from build123d import *

# Parameters (mm, degrees)
F0_W     = 0.75
F0_H     = 2
F1_DEPTH = 12
F2_W     = 6.62
F2_H     = 2
F3_DEPTH = 12
F4_DEPTH = 8
F5_W     = 8
F5_H     = 4
F6_DEPTH = 4
F7_W     = 6.62
F7_H     = 12
F8_DEPTH = 3
F9_DEPTH = 3


with BuildPart() as f1:
    # F0 (on Front) → F1 (new body, symmetric)
    with BuildSketch(Plane.XZ):
        Polygon((-4, 4), (-10, 4), (-10, -3), (10, -3), (10, 4), (4, 4), (4, 2), (4, 0), (-4, 0), (-4, 2), align=None)
        with Locations((-3.625, 3)):
            Rectangle(F0_W, F0_H)
        with Locations((3.625, 3)):
            Rectangle(F0_W, F0_H)
    extrude(amount=F1_DEPTH, both=True)

    # F2 (on Front) → F3 (cut)
    with BuildSketch(Plane.XZ):
        with Locations((0, -1)):
            Rectangle(F2_W, F2_H)
    extrude(amount=F3_DEPTH, mode=Mode.SUBTRACT)

    # F2 (on Front) → F4 (cut)
    with BuildSketch(Plane.XZ):
        with Locations((0, -1)):
            Rectangle(F2_W, F2_H)
    extrude(amount=-F4_DEPTH, mode=Mode.SUBTRACT)

    # F5 (on Top) → F6 (join)
    with BuildSketch(Plane.XY):
        with Locations((0, 10)):
            Rectangle(F5_W, F5_H)
    extrude(amount=F6_DEPTH)

    # F7 (on Top) → F8 (cut)
    with BuildSketch(Plane.XY):
        with Locations((0, -1)):
            Rectangle(F7_W, F7_H)
    extrude(amount=-F8_DEPTH, mode=Mode.SUBTRACT)

    # F6_face (on face) → F9 (join)
    with BuildSketch(Plane(origin=(0, 8, 0.988636), x_dir=(1, 0, 0), z_dir=(0, -1, 0))):
        Polygon((-4, -0.988636), (-3.31, -0.988636), (-3.31, -2.988636), (3.31, -2.988636), (3.31, -0.988636), (4, -0.988636), (4, 1.011364), (3.25, 1.011364), (3.25, 3.011364), (-3.25, 3.011364), (-3.25, 1.011364), (-4, 1.011364), align=None)
    extrude(amount=F9_DEPTH)


solid = f1.part
The model under review builds one solid part; all positions refer to its coordinate system, in mm. A direction names the side the tool comes from. Coordinates: 2 decimals unless noted, no trailing zeros. Write each loop counter-clockwise with the first axis right and the second up, starting at its lowest first coordinate (ties: lowest second). Pieces come first, ordered by that corner, then holes. Notation, with made-up numbers: M 21,-38.5 L 51,-38.5 A13 cw 51,-13.5 Z; hole C -4,42.25 d7. An arc over 180 degrees is marked long. Put each result on its own line as item: value.
1) Add section B-B on z = -0.5. Give the boundary of the cut face in (x, y).
Computed:
outline: M -10,-12 L -3.31,-12 L -3.31,5 L 3.31,5 L 3.31,-12 L 10,-12 L 10,12 L -10,12 Z
2) Draft analysis for pull direction Y (two halves, no side actions). For faces 1 (the flat face through (0, -9, -2)), 2 (the flat face through (0, -7, -2.5)), 3 (the flat face through (3.31, -3, -2)), 4 (the flat face through (0, 12, 0)), state which applies: released by +Y, released by -Y, zero draft, split by the parting line, or undercut.
Computed:
face 1: zero draft
face 2: undercut
face 3: undercut
face 4: released by +Y
3) Add section C-C on z = 3. Give the boundary of the cut face in (x, y), then the cut area to 4 significant figures.
Computed:
outline: M -10,-12 L -3.25,-12 L -3.25,5 L 3.25,5 L 3.25,-12 L 10,-12 L 10,12 L -10,12 Z
area: 369.5 mm2
4) For faces 5 (the flat face through (-4, -4, 1)), 6 (the flat face through (10, 0, 0)), 7 (the flat face through (3.25, -4, 3)), 8 (the flat face through (-0.1, -12, -2.6)), 9 (the flat face through (-3.31, -3, -2)), list the 3-axis set-ups (+Z, -Z, +X, -X, +Y, -Y) from which the entire face can be reached by the end or side of a thin tool; tool diameter is ignored.
Computed:
face 5: -Y
face 6: +Z, -Z, +X, +Y, -Y
face 7: +Z, -Y
face 8: +Z, -Z, +X, -X, -Y
face 9: none
5) Wall thickness on probe 1 along X at (y, z) = (-9.75, 3.25); probe 2 along X at (y, z) = (-2.25, -0.25); probe 3 along Z at (x, y) = (1.5, -10.5): over which ranges is each line inside the solid? List them lowest first. Write a range as [from, to].
Computed:
probe 1: x = [-10, -3.25], [3.25, 10]
probe 2: x = [-10, -3.31], [3.31, 10]
probe 3: z = [-3, -2]
6) Add section A-A on y = -6.5. Give the boundary of the cut face in (x, z).
Computed:
outline: M -10,-3 L -3.31,-3 L -3.31,0 L -4,0 L -4,2 L -3.25,2 L -3.25,4 L -10,4 Z; M 3.25,2 L 4,2 L 4,0 L 3.31,0 L 3.31,-3 L 10,-3 L 10,4 L 3.25,4 Z
7) Clearance check with a flat-ended pin moving along its axis: pin 1 Ø1.5 at (x, y) = (1, -9) entering from +Z. State where the tip first meets the part, or that it passes through.
Computed:
pin 1: stops at z = -2
